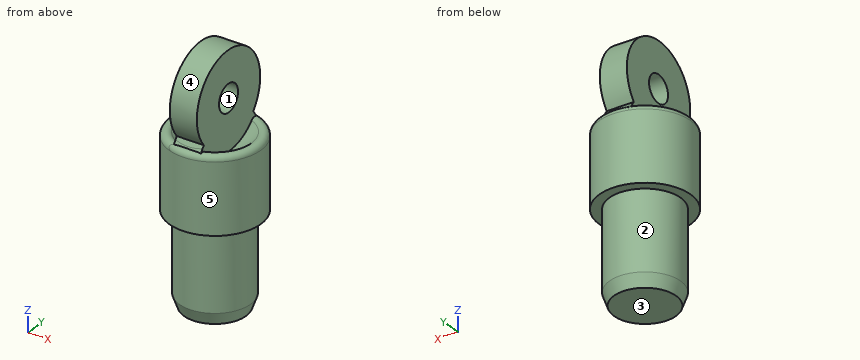
from build123d import *

# Parameters (mm, degrees)
F0_R         = 12.7
F1_DEPTH     = 25.4
F4_R         = 3.81
F5_DEPTH     = 3.81
F6_T4_ANGLE  = 90
F6_T9_ANGLE  = 90
F6_T14_ANGLE = 270
F6_T19_ANGLE = 270
F6_T24_ANGLE = 270
F6_T29_ANGLE = 270
F7_R         = 9.906
F8_DEPTH     = 25.4
F9_SIZE2     = 3.4892963227
F9_SIZE      = 1.27


# Not quite as in the source:
# - a fillet or chamfer that OpenCascade refuses, or shapes differently, is made with other operations: its cross-section is extruded or revolved along the edge and cut away or added


with BuildPart() as f1:
    # F0 (on Top) → F1 (new body)
    with BuildSketch(Plane.XY):
        Circle(F0_R)
    extrude(amount=F1_DEPTH)

    # F2 (on Right) → F3 (revolve, cut)
    with BuildSketch(Plane.YZ):
        with BuildLine():
            Line((0, 15.875), (0, 42.545))
            ThreePointArc((0, 42.545), (-13.335, 29.21), (0, 15.875))
        make_face()
    revolve(axis=Axis((0, 0, 25.198931613), (0, 0, 1)), mode=Mode.SUBTRACT)

    # F4 (on Right) → F5 (join, symmetric)
    with BuildSketch(Plane.YZ):
        with BuildLine():
            ThreePointArc((9.9246541198, 22.5559075849), (11.9860983502, 26.2819711364), (12.7, 30.48))
            ThreePointArc((12.7, 30.48), (-4.1980288636, 42.4660983502), (-9.9246541198, 22.5559075849))
            ThreePointArc((-9.9246541198, 22.5559075849), (0, 17.78), (9.9246541198, 22.5559075849))
        make_face()
        with Locations((0, 30.48)):
            Circle(F4_R, mode=Mode.SUBTRACT)
        with BuildLine():
            ThreePointArc((9.9246541198, 22.5559075849), (0, 17.78), (-9.9246541198, 22.5559075849))
            Line((-9.9246541198, 22.5559075849), (-12.0323663577, 19.4415319711))
            ThreePointArc((-12.0323663577, 19.4415319711), (-6.795833015, 14.9780300529), (0, 13.9006329783))
            ThreePointArc((0, 13.9006329783), (6.795833015, 14.9780300529), (12.0323663577, 19.4415319711))
            Line((12.0323663577, 19.4415319711), (9.9246541198, 22.5559075849))
        make_face()
    extrude(amount=F5_DEPTH, both=True)

    # F6: fillet of radius 1.524 on 2 edges, made by hand


with BuildPart() as f6_tool2:
    # F6_s3 → F6_t4 (revolve)
    with BuildSketch(Plane.XZ):
        with BuildLine():
            ThreePointArc((12.7, 19.4178140847), (11.7125077962, 20.8442555958), (10.0297435897, 20.4221408452))
            ThreePointArc((10.0297435897, 20.4221408452), (11.6075121114, 22.645863531), (12.7, 25.1440161092))
            Line((12.7, 25.1440161092), (12.7, 19.4178140847))
        make_face()
    revolve(axis=Axis((0, 0, 25.1440161092), (0, 0, -1)), revolution_arc=F6_T4_ANGLE)

    split(bisect_by=Plane.YZ.offset(3.81), keep=Keep.TOP)


with BuildPart() as f1_1:
    add(f1.part)

    # F6_t1: cut F6_tool2
    add(f6_tool2.part, mode=Mode.SUBTRACT)


with BuildPart() as f6_tool7:
    # F6_s8 → F6_t9 (revolve)
    with BuildSketch(Plane.XZ):
        with BuildLine():
            ThreePointArc((12.7, 19.4178140847), (11.7125077962, 20.8442555958), (10.0297435897, 20.4221408452))
            ThreePointArc((10.0297435897, 20.4221408452), (11.6075121114, 22.645863531), (12.7, 25.1440161092))
            Line((12.7, 25.1440161092), (12.7, 19.4178140847))
        make_face()
    revolve(axis=Axis((0, 0, 25.1440161092), (0, 0, -1)), revolution_arc=F6_T9_ANGLE)

    split(bisect_by=Plane(origin=(0, -17.2767572385, 11.6923702143), x_dir=(1, 0, 0), z_dir=(0, -0.8281687795, 0.5604787887)), keep=Keep.TOP)


with BuildPart() as f1_2:
    add(f1_1.part)

    # F6_t6: cut F6_tool7
    add(f6_tool7.part, mode=Mode.SUBTRACT)


with BuildPart() as f6_tool12:
    # F6_s13 → F6_t14 (revolve)
    with BuildSketch(Plane.YZ):
        with BuildLine():
            ThreePointArc((-12.7, 19.4178140847), (-11.7125077962, 20.8442555958), (-10.0297435897, 20.4221408452))
            ThreePointArc((-10.0297435897, 20.4221408452), (-11.6075121114, 22.645863531), (-12.7, 25.1440161092))
            Line((-12.7, 25.1440161092), (-12.7, 19.4178140847))
        make_face()
    revolve(axis=Axis((0, 0, 25.1440161092), (0, 0, -1)), revolution_arc=F6_T14_ANGLE)

    split(bisect_by=Plane(origin=(0, -17.2767572385, 11.6923702143), x_dir=(1, 0, 0), z_dir=(0, -0.8281687795, 0.5604787887)), keep=Keep.TOP)


with BuildPart() as f1_3:
    add(f1_2.part)

    # F6_t11: cut F6_tool12
    add(f6_tool12.part, mode=Mode.SUBTRACT)


with BuildPart() as f6_tool17:
    # F6_s18 → F6_t19 (revolve)
    with BuildSketch(Plane.YZ):
        with BuildLine():
            ThreePointArc((-12.7, 19.4178140847), (-11.7125077962, 20.8442555958), (-10.0297435897, 20.4221408452))
            ThreePointArc((-10.0297435897, 20.4221408452), (-11.6075121114, 22.645863531), (-12.7, 25.1440161092))
            Line((-12.7, 25.1440161092), (-12.7, 19.4178140847))
        make_face()
    revolve(axis=Axis((0, 0, 25.1440161092), (0, 0, -1)), revolution_arc=F6_T19_ANGLE)

    split(bisect_by=Plane.YZ.offset(-3.81), keep=Keep.BOTTOM)


with BuildPart() as f1_4:
    add(f1_3.part)

    # F6_t16: cut F6_tool17
    add(f6_tool17.part, mode=Mode.SUBTRACT)


with BuildPart() as f6_tool22:
    # F6_s23 → F6_t24 (revolve)
    with BuildSketch(Plane.YZ):
        with BuildLine():
            ThreePointArc((-12.7, 19.4178140847), (-11.7125077962, 20.8442555958), (-10.0297435897, 20.4221408452))
            ThreePointArc((-10.0297435897, 20.4221408452), (-11.6075121114, 22.645863531), (-12.7, 25.1440161092))
            Line((-12.7, 25.1440161092), (-12.7, 19.4178140847))
        make_face()
    revolve(axis=Axis((0, 0, 25.1440161092), (0, 0, -1)), revolution_arc=F6_T24_ANGLE)

    split(bisect_by=Plane.YZ.offset(3.81), keep=Keep.TOP)


with BuildPart() as f1_5:
    add(f1_4.part)

    # F6_t21: cut F6_tool22
    add(f6_tool22.part, mode=Mode.SUBTRACT)


with BuildPart() as f6_tool27:
    # F6_s28 → F6_t29 (revolve)
    with BuildSketch(Plane.YZ):
        with BuildLine():
            ThreePointArc((-12.7, 19.4178140847), (-11.7125077962, 20.8442555958), (-10.0297435897, 20.4221408452))
            ThreePointArc((-10.0297435897, 20.4221408452), (-11.6075121114, 22.645863531), (-12.7, 25.1440161092))
            Line((-12.7, 25.1440161092), (-12.7, 19.4178140847))
        make_face()
    revolve(axis=Axis((0, 0, 25.1440161092), (0, 0, -1)), revolution_arc=F6_T29_ANGLE)

    split(bisect_by=Plane(origin=(0, 17.2767572385, 11.6923702143), x_dir=(1, 0, 0), z_dir=(0, 0.8281687795, 0.5604787887)), keep=Keep.TOP)


with BuildPart() as f1_6:
    add(f1_5.part)

    # F6_t26: cut F6_tool27
    add(f6_tool27.part, mode=Mode.SUBTRACT)

    # F7 (on face) → F8 (join)
    with BuildSketch(Plane(origin=(0, 0, 0), x_dir=(1, 0, 0), z_dir=(0, 0, -1))):
        Circle(F7_R)
    extrude(amount=F8_DEPTH)

    # F9
    f9_edges = [f1_6.edges().sort_by_distance(p)[0] for p in [
        (-9.906, 0, -25.4),
    ]]
    f9_side = f1_6.faces().sort_by_distance((0, 0, -25.4))[0]
    chamfer(f9_edges, length=F9_SIZE, length2=F9_SIZE2, reference=f9_side)


solid = f1_6.part
Here's how the part is built. I have some questions about the finished solid (model axes, mm). Face numbers are marked on the shaded views. A direction names the side the tool comes from. Coordinates: 2 decimals unless noted, no trailing zeros. Write each loop counter-clockwise with the first axis right and the second up, starting at its lowest first coordinate (ties: lowest second). Pieces come first, ordered by that corner, then holes.
Item 1: I want a section at D-D on z = -12. Write out the boundary of the cut face in (x, y).
Item 2: I want a section at B-B on x = 0. Write out the boundary of the cut face in (y, z), and give its area (3 significant figures).
Item 3: I want a section at C-C on z = 18.5. Write out the boundary of the cut face in (x, y), and give its area (3 significant figures).
Item 4: If we mould it in two halves opening along Z, with no side actions, what happens to the marked faces 3, 4 and 5? For each: +Z half, -Z half, draft (parallel to the pull), parting line (faces both ways), or undercut.
Item 5: If I drill on line 1 (Z direction, x = -0.5, y = 0); line 2 (Z direction, x = 1, y = 10.25); line 3 (X direction, y = -2, z = 34), over which ranges is the centre line in solid material (lowest first)?
Item 6: On a 3-axis mill with a long thin cutter (end or side, diameter ignored), from which of +Z, -Z, +X, -X, +Y, -Y can I reach the whole of each face in a straight line? I mean the marked faces 1 and 2. Say none if no direction works.
Item 7: Will these pins go through, and if not, where does the flat tip stop? pin 1 (12.5 mm diameter, centred on y = -0.5, z = 26, fed in from +X); pin 2 (3 mm diameter, centred on y = -5, z = 35.5, fed in from +X); pin 3 (1.5 mm diameter, centred on y = 1.5, z = 21, fed in from +X).
Item 8: I want a section at A-A on z = 30.48. Write out the boundary of the cut face in (x, y).
Findings below:
1. outline: circle Ø19.81 at (0, 0)
2. outline: (-12.7, 0) - (-9.91, 0) - (-9.91, -21.91) - (-8.64, -25.4) - (8.64, -25.4) - (9.91, -21.91) - (9.91, 0) - (12.7, 0) - (12.7, 19.42) arc R1.52 ccw to (11.02, 20.93) - (9.92, 22.56) arc R12.7 ccw (long way) to (-9.92, 22.56) - (-11.02, 20.93) arc R1.52 ccw to (-12.7, 19.42) - close; hole circle Ø7.62 at (0, 30.48)
2. area: 1,460 mm2
3. outline: circle Ø25.4 at (0, 0); hole (-3.81, -6.97) - (-3.81, 6.97) arc R7.94 ccw to start; hole (3.81, -6.97) arc R7.94 ccw to (3.81, 6.97) - close
3. area: 425 mm2
4. face 3: -Z half
4. face 4: undercut
4. face 5: draft
5. line 1: z = -25.4 to 26.67, 34.29 to 43.18
5. line 2: z = 0 to 22.08, 22.98 to 37.98
5. line 3: x = -3.81 to 3.81
6. face 1: +X, -X
6. face 2: -Z
7. pin 1: stops at x = 12.66
7. pin 2: stops at x = 3.81
7. pin 3: stops at x = 12.37
8. outline: (-3.81, -12.7) - (3.81, -12.7) - (3.81, -3.81) - (-3.81, -3.81) - close; (-3.81, 3.81) - (3.81, 3.81) - (3.81, 12.7) - (-3.81, 12.7) - close
